```python
from build123d import *

# Parameters (mm, degrees)
SKETCH_1_R      = 2.6
EXTRUDE_1_DEPTH = 2
SKETCH_2_R      = 2.6
EXTRUDE_2_DEPTH = 2
EXTRUDE_3_DEPTH = 16


with BuildPart() as part:
    # Sketch 1 → Extrude 1 (new body)
    with BuildSketch(Plane.XY):
        with BuildLine():
            Line((-8, 32), (-8, 0))
            Line((-8, 0), (8, 0))
            Line((8, 0), (8, 32))
            ThreePointArc((8, 32), (0, 40), (-8, 32))
        make_face()
        with Locations((0, 32)):
            Circle(SKETCH_1_R, mode=Mode.SUBTRACT)
        with Locations((0, 14)):
            Circle(SKETCH_1_R, mode=Mode.SUBTRACT)
    extrude(amount=EXTRUDE_1_DEPTH)



with BuildPart() as body_2:
    # Sketch 2 → Extrude 2 (new body)
    with BuildSketch(Plane(origin=(0, 0, 0), x_dir=(1, 0, 0), z_dir=(0, 1, 0))):
        with BuildLine():
            Line((-8, 32), (-8, 0))
            Line((-8, 0), (8, 0))
            Line((8, 0), (8, 32))
            ThreePointArc((8, 32), (0, 40), (-8, 32))
        make_face()
        with Locations((0, 32)):
            Circle(SKETCH_2_R, mode=Mode.SUBTRACT)
        with Locations((0, 14)):
            Circle(SKETCH_2_R, mode=Mode.SUBTRACT)
    extrude(amount=-EXTRUDE_2_DEPTH)


with BuildPart() as part_1:
    add(part.part)

    add(body_2.part)  # Extrude 3 merges body 2
    # Sketch 3 → Extrude 3 (add)
    with BuildSketch(Plane(origin=(8, 0, 0), x_dir=(0, 0, -1), z_dir=(1, 0, 0))):
        Polygon((0, 0), (0, -2), (-2, 0), align=None)
    extrude(amount=-EXTRUDE_3_DEPTH)


solid = part_1.part
```
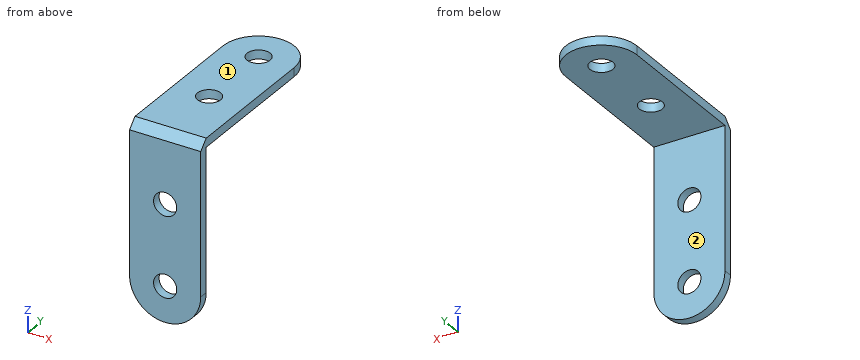
Part model, mm, in its own coordinate system. Face numbers are marked on the shaded views. A direction names the side the tool comes from. Coordinates: 2 decimals unless noted, no trailing zeros. Write each loop counter-clockwise with the first axis right and the second up, starting at its lowest first coordinate (ties: lowest second). Pieces come first, ordered by that corner, then holes.
Item 1: Slice it at B-B (y = 14). Write the cut outline in (x, z).
Item 2: Probe line 1 (Z direction, x = 0, y = -0.7); line 2 (X direction, y = -1.4, z = -32); line 3 (Y direction, x = 0, z = 0.9). List the from-to ranges inside material, lowest first.
Item 3: Slice it at D-D (x = 6.75). Write the cut outline in (y, z).
Item 4: Pin check, flat tips, straight feed: pin 1 (4.5 mm diameter, centred on x = 0, y = 14, fed in from +Z); pin 2 (8 mm diameter, centred on y = 2.5, z = -28, fed in from +X); pin 3 (1 mm diameter, centred on x = 0.5, y = 23.5, fed in from -Z); pin 4 (8 mm diameter, centred on x = -5.5, z = -13, fed in from +Y). Stop position of each tip, or through.
Item 5: Which spindle directions (+Z, -Z, +X, -X, +Y, -Y) get a long thin tool onto all of the face, cutting with end or side? Do the marked faces 1 and 2. Say none if no direction does.
Item 6: Slice it at C-C (x = 0.5). Write the cut outline in (y, z), and give its area (3 significant figures).
Item 7: Slice it at A-A (z = -14). Write the cut outline in (x, y), and give its area (3 significant figures).
Results found:
1. outline: (-8, 0) - (-2.6, 0) - (-2.6, 2) - (-8, 2) - close; (2.6, 0) - (8, 0) - (8, 2) - (2.6, 2) - close
2. line 1: z = -40 to -34.6, -29.4 to -16.6, -11.4 to 1.3
2. line 2: x = -8 to -2.6, 2.6 to 8
2. line 3: y = -1.1 to 11.4, 16.6 to 29.4, 34.6 to 40
3. outline: (-2, -36.29) - (0, -36.29) - (0, 0) - (36.29, 0) - (36.29, 2) - (0, 2) - (-2, 0) - close
4. pin 1: passes through
4. pin 2: stops at x = 8
4. pin 3: stops at z = 0
4. pin 4: stops at y = 0
5. face 1: +Z, +X, -X, +Y, -Y
5. face 2: -Z, +X, -X, +Y
6. outline: (-2, -39.98) - (0, -39.98) - (0, -34.55) - (-2, -34.55) - close; (-2, -29.45) - (0, -29.45) - (0, -16.55) - (-2, -16.55) - close; (-2, -11.45) - (0, -11.45) - (0, 0) - (11.45, 0) - (11.45, 2) - (0, 2) - (-2, 0) - close; (16.55, 0) - (29.45, 0) - (29.45, 2) - (16.55, 2) - close; (34.55, 0) - (39.98, 0) - (39.98, 2) - (34.55, 2) - close
6. area: 121 mm2
7. outline: (-8, -2) - (-2.6, -2) - (-2.6, 0) - (-8, 0) - close; (2.6, -2) - (8, -2) - (8, 0) - (2.6, 0) - close
7. area: 21.6 mm2
